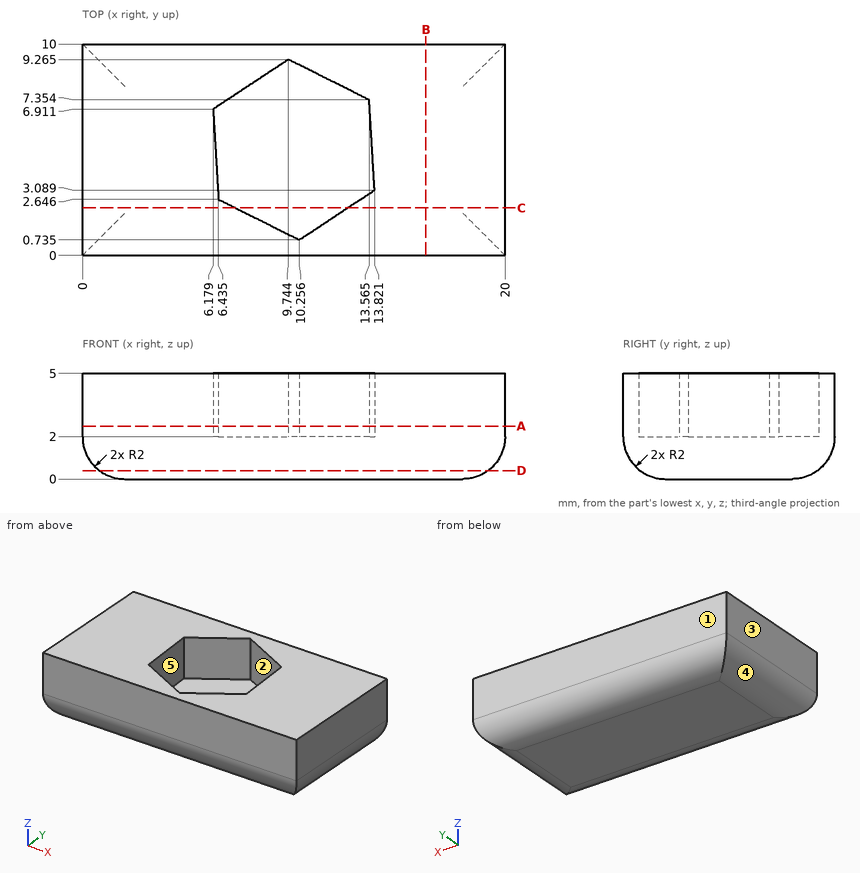
Can you work these out from the drawing? Everything is in mm from the part's minimum corner. A direction names the side the tool comes from. Give positions to 0.01 mm unless a question says otherwise; leave off trailing zeros. Loops run counter-clockwise (first coordinate to the right, second up) from the corner with the lowest first, then second, coordinate; pieces in that order, holes last. Notation, with made-up numbers: (-7.75, 81.5) -> (25.25, 81.5) arc R11 ccw to (25.25, 97.5) -> close; hole circle Ø6 at (-31, -33.5). An arc over 180 degrees is marked (long way). Write item = value, one per line.
1) Suppose I cut it at D-D on z = 0.4. Write out the boundary of the cut face in (x, y).
Check result:
outline = (0.8, 0.8) -> (19.2, 0.8) -> (19.2, 9.2) -> (0.8, 9.2) -> close
2) For the marked faces 4 and 5, which set-ups out of +Z, -Z, +X, -X, +Y, -Y let a thin tool reach every point of the face, with its end or its side?
Check result:
face_4 = -Z, -X, +Y, -Y
face_5 = +Z
3) Will these pins go through, and if not, where does the flat tip stop? pin 1 (1 mm diameter, centred on y = 1, z = 1, fed in from +X); pin 2 (2.5 mm diameter, centred on x = 11.5, y = 5.5, fed in from +Z).
Check result:
pin_1 = 19.94
pin_2 = 2
4) Suppose I cut it at C-C on y = 2.25. Write out the boundary of the cut face in (x, z).
Check result:
outline = (0, 2) arc R2 ccw to (2, 0) -> (18, 0) arc R2 ccw to (20, 2) -> (20, 5) -> (12.55, 5) -> (12.55, 2) -> (7.23, 2) -> (7.23, 5) -> (0, 5) -> close
5) Suppose I cut it at B-B on x = 16.25. Write out the boundary of the cut face in (y, z), then the cut area to 3 significant figures.
Check result:
outline = (0, 2) arc R2 ccw to (2, 0) -> (8, 0) arc R2 ccw to (10, 2) -> (10, 5) -> (0, 5) -> close
area = 48.3 mm2
6) I need wall thicknesses on L1, parallel to Y at x = 2, z = 1.9; L2, parallel to Z at x = 12.75, y = 6.5; L3, parallel to X at y = 6.5, z = 4.25. Which ranges of each line are inside material? Lowest first, please. Write a range as from..to.
Check result:
L1 = 0..10
L2 = 0..2
L3 = 0..6.2, 13.62..20
7) Suppose I cut it at A-A on z = 2.5. Write out the boundary of the cut face in (x, y) (1 decimal).
Check result:
outline = (0, 0) -> (20, 0) -> (20, 10) -> (0, 10) -> close; hole (6.2, 6.9) -> (6.4, 2.6) -> (10.3, 0.7) -> (13.8, 3.1) -> (13.6, 7.4) -> (9.7, 9.3) -> close
8) Thinking about a two-plate mould opening in Y: for the marked faces 1, 2 and 3, which applies, released by +Y, released by -Y, zero draft, split by the parting line, or undercut?
Check result:
face_1 = released by +Y
face_2 = undercut
face_3 = zero draft
